Input: part model. Units: mm. Frame: model coordinates. Face numbers are marked on the shaded views. A direction names the side the tool comes from. Coordinates: 2 decimals unless noted, no trailing zeros. Order: outer loops, then holes, each group sorted by start corner. A loop starts at its lowest first (then second) coordinate and runs counter-clockwise, first axis right, second up. Notation, with made-up numbers: (4.25, 39.25) -> (10.25, 39.25) arc R17 cw to (10.25, 70.25) -> close; hole circle Ø1 at (44.25, 42). An arc over 180 degrees is marked (long way). Use CSV: the item, a comma, the result in double quotes. Start each with the question number.
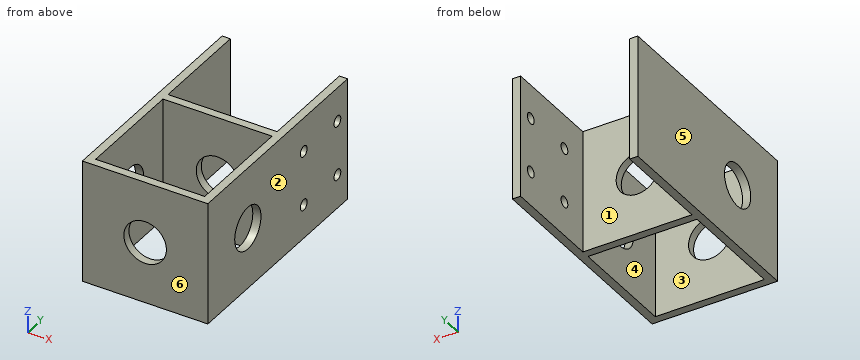
```python
from build123d import *

# Parameters (mm, degrees)
SKETCH1_W           = 46
SKETCH1_H           = 45
BOSS_EXTRUDE1_DEPTH = 3
SKETCH5_W           = 3
SKETCH5_H           = 45
BOSS_EXTRUDE3_DEPTH = 35
SKETCH9_R           = 7.8
CUT_EXTRUDE5_DEPTH  = 10
SKETCH11_R          = 7.8
CUT_EXTRUDE8_DEPTH  = 47
SKETCH12_W          = 3
SKETCH12_H          = 45
BOSS_EXTRUDE4_DEPTH = 45
SKETCH13_R          = 2
CUT_EXTRUDE9_DEPTH  = 10


with BuildPart() as part:
    # Sketch1 → Boss-Extrude1 (new body)
    with BuildSketch(Plane(origin=(0, 0, 0), x_dir=(1, 0, 0), z_dir=(0, 1, 0))):
        Rectangle(SKETCH1_W, SKETCH1_H)
    boss_extrude1 = extrude(amount=BOSS_EXTRUDE1_DEPTH)

    # Sketch5 → Boss-Extrude3 (add)
    with BuildSketch(Plane(origin=(0, 3, 0), x_dir=(1, 0, 0), z_dir=(0, 1, 0))):
        with Locations((21.5, 0)):
            Rectangle(SKETCH5_W, SKETCH5_H)
        with Locations((-21.5, 0)):
            Rectangle(SKETCH5_W, SKETCH5_H)
    extrude(amount=BOSS_EXTRUDE3_DEPTH)

    # Sketch9 → Cut-Extrude5 (cut)
    with BuildSketch(Plane(origin=(0, 3, 0), x_dir=(1, 0, 0), z_dir=(0, 1, 0))):
        Circle(SKETCH9_R)
    cut_extrude5 = extrude(amount=-CUT_EXTRUDE5_DEPTH, mode=Mode.SUBTRACT)

    # Sketch11 → Cut-Extrude8 (cut, through all)
    with BuildSketch(Plane.ZY.offset(23)):
        with Locations((0, 23.75)):
            Circle(SKETCH11_R)
    extrude(amount=-CUT_EXTRUDE8_DEPTH, mode=Mode.SUBTRACT)

    # Sketch12 → Boss-Extrude4 (add)
    with BuildSketch(Plane(origin=(0, 38, 0), x_dir=(1, 0, 0), z_dir=(0, 1, 0))):
        with Locations((-21.5, 0)):
            Rectangle(SKETCH12_W, SKETCH12_H)
        with Locations((21.5, 0)):
            Rectangle(SKETCH12_W, SKETCH12_H)
    extrude(amount=BOSS_EXTRUDE4_DEPTH)

    # Sketch13 → Cut-Extrude9 (cut)
    with BuildSketch(Plane(origin=(23, 0, 0), x_dir=(0, 0, -1), z_dir=(1, 0, 0))):
        with Locations((-10, 76.955662999)):
            Circle(SKETCH13_R)
        with Locations((10, 76.955662999)):
            Circle(SKETCH13_R)
        with Locations((10, 56.955662999)):
            Circle(SKETCH13_R)
        with Locations((-10, 56.955662999)):
            Circle(SKETCH13_R)
    extrude(amount=-CUT_EXTRUDE9_DEPTH, mode=Mode.SUBTRACT)

    # Mirror1: Boss-Extrude1, Cut-Extrude5 across plane
    add(boss_extrude1.mirror(Plane.ZX.offset(23)))
    add(cut_extrude5.mirror(Plane.ZX.offset(23)), mode=Mode.SUBTRACT)


solid = part.part
```
1. Pull-direction query (X, two-part tool) for the marked faces 4, 5 and 6; classes: released by +X, released by -X, zero draft, split by the parting line, or undercut.
2. Access query for the marked faces 1, 2 and 3. Directions: +Z, -Z, +X, -X, +Y, -Y. A direction counts if a zero-diameter tool reaches every point of the face in a straight line with its end or side. Return the directions, or none.
3. Contact query for flat-ended pins moving along their axis: P1, Ø3.5, axis at y = 56.96, z = -10, coming from the +X side; P2, Ø12, axis at x = 3.5, z = 0, coming from the +Y side. Output: stop coordinate, or through.
4. Section A-A on x = 18. Return loops of the section in (y, z).
5. Material intervals for line 1 along Y through (x, z) = (21, 10); line 2 along Y through (x, z) = (6.5, 12); line 3 along X through (y, z) = (45, 0), sorted ascending.
6. Section C-C on y = 23.75. Return loops of the section in (x, z), then the cut area to 3 significant figures.
7. Section B-B on z = 10. Return loops of the section in (x, y).
8. Section D-D on y = 72. Return loops of the section in (x, z), then the cut area to 3 significant figures.
Values follow:
1,face 4,"undercut"
1,face 5,"released by -X"
1,face 6,"zero draft"
2,face 1,"+Z, -Z, +Y"
2,face 2,"+Z, -Z, +X, +Y, -Y"
2,face 3,"+Z, -Z"
3,P1,"stops at x = -20"
3,P2,"stops at y = 46"
4,outline,"(0, -22.5) -> (3, -22.5) -> (3, 22.5) -> (0, 22.5) -> close; (43, -22.5) -> (46, -22.5) -> (46, 22.5) -> (43, 22.5) -> close"
5,line 1,"y = 0 to 54.96, 58.96 to 74.96, 78.96 to 83"
5,line 2,"y = 0 to 3, 43 to 46"
5,line 3,"x = -23 to -7.8, 7.8 to 23"
6,outline,"(-23, -22.5) -> (-20, -22.5) -> (-20, -7.8) -> (-23, -7.8) -> close; (-23, 7.8) -> (-20, 7.8) -> (-20, 22.5) -> (-23, 22.5) -> close; (20, -22.5) -> (23, -22.5) -> (23, -7.8) -> (20, -7.8) -> close; (20, 7.8) -> (23, 7.8) -> (23, 22.5) -> (20, 22.5) -> close"
6,area,"176 mm2"
7,outline,"(-23, 0) -> (23, 0) -> (23, 54.96) -> (20, 54.96) -> (20, 46) -> (-20, 46) -> (-20, 83) -> (-23, 83) -> close; (20, 58.96) -> (23, 58.96) -> (23, 74.96) -> (20, 74.96) -> close; (20, 78.96) -> (23, 78.96) -> (23, 83) -> (20, 83) -> close; hole (-20, 3) -> (20, 3) -> (20, 43) -> (-20, 43) -> close"
8,outline,"(-23, -22.5) -> (-20, -22.5) -> (-20, 22.5) -> (-23, 22.5) -> close; (20, -22.5) -> (23, -22.5) -> (23, 22.5) -> (20, 22.5) -> close"
8,area,"270 mm2"
